Can you work these out from the drawing? Everything is in mm from the part's minimum corner. A direction names the side the tool comes from. Coordinates: 2 decimals unless noted, no trailing zeros. Loops run counter-clockwise (first coordinate to the right, second up) from the corner with the lowest first, then second, coordinate; pieces in that order, holes last.
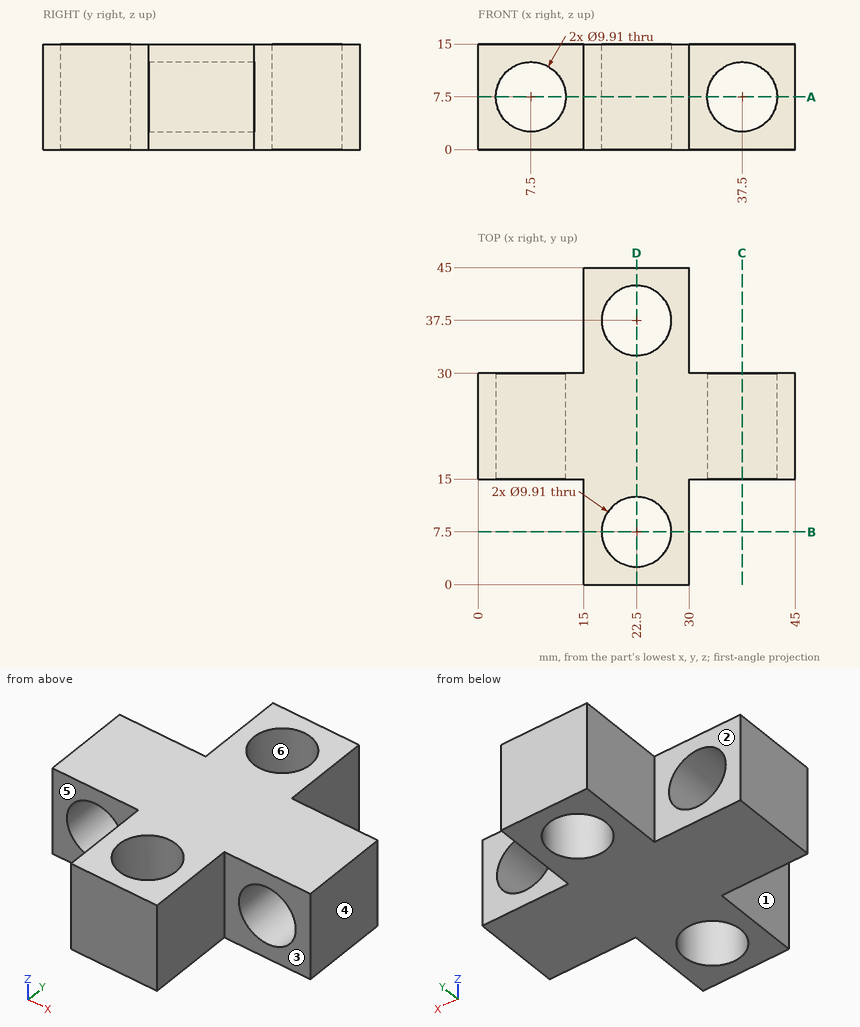
1. We'd pull the mould along X, two halves only. Please class the marked faces 4, 5 and 6: +X half, -X half, draft (parallel to the pull), parting line (faces both ways), or undercut.
2. On a 3-axis mill with a long thin cutter (end or side, diameter ignored), from which of +Z, -Z, +X, -X, +Y, -Y can I reach the whole of each face in a straight line? I mean the marked faces 1, 2 and 3. Say none if no direction works.
3. I need wall thicknesses on line 1 along Z through (x, y) = (7.5, 20) (3 decimals); line 2 along Y through (x, z) = (22.5, 12.25) (3 decimals); line 3 along Y through (x, z) = (19.5, 7.75). Which ranges of each line are inside material? Lowest first, please.
4. For pin 1 (2 mm diameter, centred on y = 9, z = 13, fed in from -X); pin 2 (12 mm diameter, centred on x = 7.5, y = 37.5, fed in from +Z); pin 3 (5 mm diameter, centred on x = 40, y = 17.5, fed in from -Z); pin 4 (4.5 mm diameter, centred on x = 5.5, z = 5.5, fed in from +Y), each with a flat end and sliding along its axis, tell me the tip position at first contact or that it passes through.
5. I want a section at C-C (x = 37.5). Please give me the cut outline in (y, z) (3 decimals).
6. I want a section at B-B (y = 7.5). Please give me the cut outline in (x, z) (3 decimals).
7. I want a section at D-D (x = 22.5). Please give me the cut outline in (y, z) (3 decimals).
8. I want a section at A-A (z = 7.5). Please give me the cut outline in (x, y) (3 decimals).
Response values:
1. face 4: +X half
1. face 5: draft
1. face 6: undercut
2. face 1: +Z, -Z, -X, -Y
2. face 2: +Z, -Z, -X, +Y
2. face 3: +Z, -Z, +X, -Y
3. line 1: z = 0 to 2.545, 12.455 to 15
3. line 2: y = 0 to 2.545, 12.455 to 32.545, 42.455 to 45
3. line 3: y = 0 to 3.56, 11.44 to 33.56, 41.44 to 45
4. pin 1: stops at x = 15
4. pin 2: passes through
4. pin 3: stops at z = 0
4. pin 4: stops at y = 30
5. outline: (15, 0) - (30, 0) - (30, 2.545) - (15, 2.545) - close; (15, 12.455) - (30, 12.455) - (30, 15) - (15, 15) - close
6. outline: (15, 0) - (17.545, 0) - (17.545, 15) - (15, 15) - close; (27.455, 0) - (30, 0) - (30, 15) - (27.455, 15) - close
7. outline: (0, 0) - (2.545, 0) - (2.545, 15) - (0, 15) - close; (12.455, 0) - (32.545, 0) - (32.545, 15) - (12.455, 15) - close; (42.455, 0) - (45, 0) - (45, 15) - (42.455, 15) - close
8. outline: (0, 15) - (2.545, 15) - (2.545, 30) - (0, 30) - close; (12.455, 15) - (15, 15) - (15, 0) - (30, 0) - (30, 15) - (32.545, 15) - (32.545, 30) - (30, 30) - (30, 45) - (15, 45) - (15, 30) - (12.455, 30) - close; (42.455, 15) - (45, 15) - (45, 30) - (42.455, 30) - close; hole circle Ø9.91 at (22.5, 7.5); hole circle Ø9.91 at (22.5, 37.5)
